Input: part model. Units: mm. Frame: model coordinates. A direction names the side the tool comes from. Give positions to 0.01 mm unless a question says otherwise; leave off trailing zeros. Write each loop counter-clockwise with the first axis right and the second up, starting at its lowest first coordinate (ties: lowest second). Pieces come first, ordered by that corner, then holes. Notation, with made-up numbers: (55.25, -5) - (93.25, -5) arc R32 ccw to (93.25, 23) - close; hole circle Ø11 at (76.25, 17). An arc over 180 degrees is marked (long way). Use a Markdown table: item, result. Add a question column.
1. Section query D-D, the plane x = 2.5. Return loops of the section in (y, z).
2. Section query C-C, the plane x = 0. Return loops of the section in (y, z), plus the area to 3 significant figures.
3. Set-up query: faces 3 (the cylindrical face through (1.53, 4.76, 10.33)), 4 (the cylindrical face through (-1.606, -4.74, 10.328)), 5 (the cylindrical face through (0, 3, 10)). Return all of +Z, -Z, +X, -X, +Y, -Y with unobstructed straight access to the full face (end or side cutting, diameter ignored); none if empty.
4. Pin query (flat end, axial travel): pin 1 (1.5 mm diameter, centred on x = -2.5, z = 9, fed in from -Y); pin 2 (1.5 mm diameter, centred on x = -4, z = 4, fed in from -Y); pin 3 (5 mm diameter, centred on x = -2, y = -0.5, fed in from +Z). Return the tip coordinate at first contact, or that it passes through.
5. Material intervals for probe 1 along Y at (x, z) = (0, 2.5); probe 2 along Z at (x, y) = (-6.5, 0), sorted ascending.
6. Section query B-B, the plane z = 9. Return loops of the section in (x, y) (3 decimals).
7. Section query A-A, the plane y = 0. Return loops of the section in (x, z), plus the area to 3 significant figures.
8. Mould query, pull axis Y, two halves, no side actions, for faces 1 (the cylindrical face through (-2.476, 4.414, 10.328)), 2 (the flat face through (1.5, 0.1, 0)). Classes: released by +Y, released by -Y, zero draft, split by the parting line, or undercut.
```python
from build123d import *

# Parameters (mm, degrees)
F0_R     = 7
F1_DEPTH = 7
F3_DEPTH = 6.75
F4_R     = 3
F5_DEPTH = 6.75
F6_R     = 1
F7_DEPTH = 13.751


with BuildPart() as f1:
    # F0 (on Top) → F1 (new body)
    with BuildSketch(Plane.XY):
        Circle(F0_R)
    extrude(amount=F1_DEPTH)

    # F2 (on face) → F3 (join)
    with BuildSketch(Plane.XY.offset(7)):
        with BuildLine():
            ThreePointArc((2.9875473685, 0.273058091), (2.2988535655, 1.9275041594), (0.7898544942, 2.8941544323))
            ThreePointArc((0.7898544942, 2.8941544323), (-0.273058091, 2.9875473685), (-1.3014286637, 2.7030137686))
            ThreePointArc((-1.3014286637, 2.7030137686), (-2.6101876905, 1.4788239315), (-2.9875473685, -0.273058091))
            Line((-2.9875473685, -0.273058091), (2.9875473685, 0.273058091))
        make_face()
        with BuildLine():
            ThreePointArc((-1.3014286637, 2.7030137686), (-0.273058091, 2.9875473685), (0.7898544942, 2.8941544323))
            ThreePointArc((0.7898544942, 2.8941544323), (1.5438295644, 4.7878332543), (2.7289268388, 6.4461584148))
            ThreePointArc((2.7289268388, 6.4461584148), (-0.7171765928, 6.9631643478), (-3.9855530681, 5.7545952717))
            ThreePointArc((-3.9855530681, 5.7545952717), (-2.4574856727, 4.3924118424), (-1.3014286637, 2.7030137686))
        make_face()
        with BuildLine():
            ThreePointArc((3, 0), (2.9968852252, 0.1366709452), (2.9875473685, 0.273058091))
            Line((2.9875473685, 0.273058091), (-2.9875473685, -0.273058091))
            ThreePointArc((-2.9875473685, -0.273058091), (-2.2988535655, -1.9275041594), (-0.7898544942, -2.8941544323))
            ThreePointArc((-0.7898544942, -2.8941544323), (0.273058091, -2.9875473685), (1.3014286637, -2.7030137686))
            ThreePointArc((1.3014286637, -2.7030137686), (2.5401068867, -1.5962008033), (3, 0))
        make_face()
        with BuildLine():
            ThreePointArc((1.3014286637, -2.7030137686), (0.273058091, -2.9875473685), (-0.7898544942, -2.8941544323))
            ThreePointArc((-0.7898544942, -2.8941544323), (-1.6204974061, -4.7651343928), (-2.8763053334, -6.3817605431))
            ThreePointArc((-2.8763053334, -6.3817605431), (0.5570104085, -6.9778033366), (3.8522907412, -5.8446433634))
            ThreePointArc((3.8522907412, -5.8446433634), (2.3862030644, -4.4286331899), (1.3014286637, -2.7030137686))
        make_face()
    extrude(amount=F3_DEPTH)

    # F4 (on face) → F5 (cut)
    with BuildSketch(Plane.XY.offset(13.75)):
        Circle(F4_R)
    extrude(amount=-F5_DEPTH, mode=Mode.SUBTRACT)

    # F6 (on face) → F7 (cut, through all)
    with BuildSketch(Plane(origin=(0, 0, 0), x_dir=(1, 0, 0), z_dir=(0, 0, -1))):
        Circle(F6_R)
    extrude(amount=-F7_DEPTH, mode=Mode.SUBTRACT)


solid = f1.part
```
Result sheet:
| question | item | result |
|---|---|---|
| 1 | outline | (-6.54, 0) - (6.54, 0) - (6.54, 13.75) - (6.19, 13.75) - (6.19, 7) - (-4.57, 7) - (-4.57, 13.75) - (-6.54, 13.75) - close |
| 2 | outline | (-7, 0) - (-1, 0) - (-1, 7) - (-3, 7) - (-3, 13.75) - (-7, 13.75) - close; (1, 0) - (7, 0) - (7, 13.75) - (3, 13.75) - (3, 7) - (1, 7) - close |
| 2 | area | 138 mm² |
| 3 | face 3 | +Z, +X |
| 3 | face 4 | +Z, -X |
| 3 | face 5 | +Z |
| 4 | pin 1 | stops at y = -6.78 |
| 4 | pin 2 | stops at y = -6.2 |
| 4 | pin 3 | stops at z = 7 |
| 5 | probe 1 | y = -7 to -1, 1 to 7 |
| 5 | probe 2 | z = 0 to 7 |
| 6 | outline | (-3.986, 5.755) arc R8.458 cw to (-1.301, 2.703) arc R3 cw to (0.79, 2.894) arc R8.458 cw to (2.729, 6.446) arc R7 ccw to start; (-2.876, -6.382) arc R7 ccw to (3.852, -5.845) arc R8.458 cw to (1.301, -2.703) arc R3 cw to (-0.79, -2.894) arc R8.458 cw to start |
| 7 | outline | (-7, 0) - (-1, 0) - (-1, 7) - (-7, 7) - close; (1, 0) - (7, 0) - (7, 7) - (1, 7) - close |
| 7 | area | 84.0 mm² |
| 8 | face 1 | undercut |
| 8 | face 2 | zero draft |
